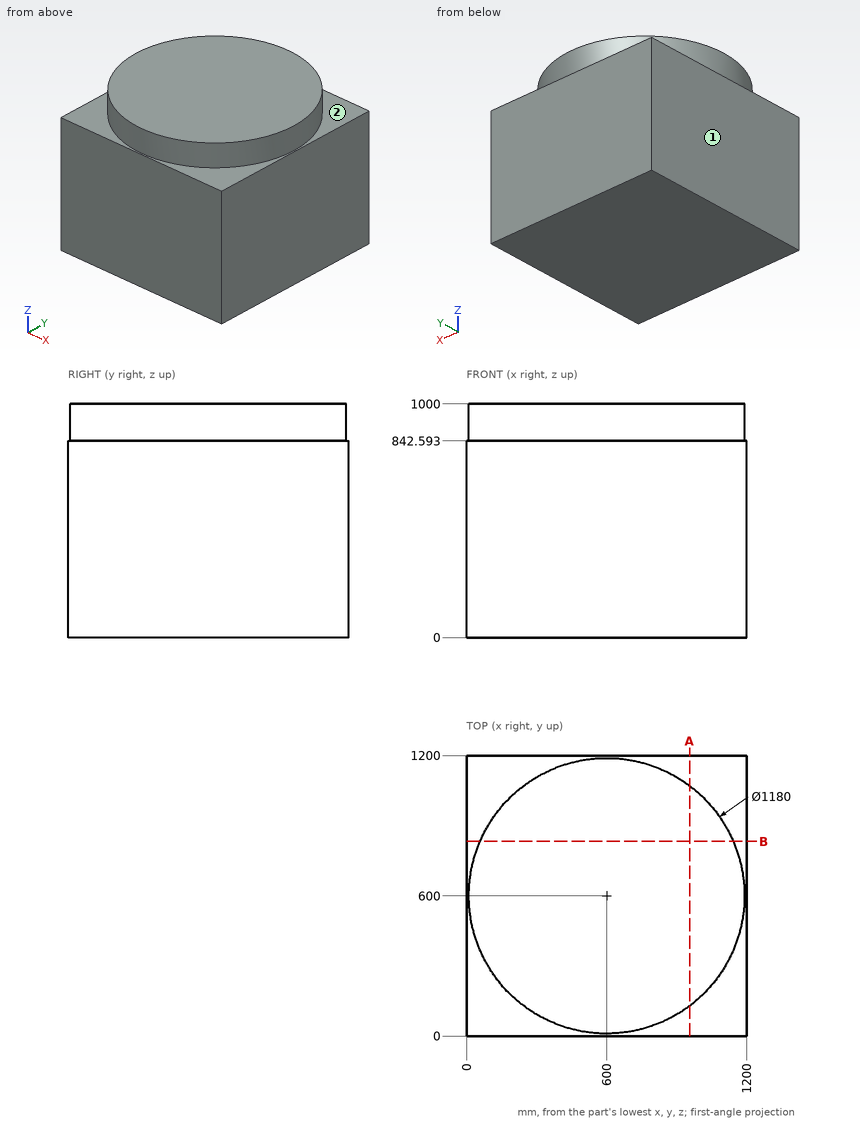
Answer from the drawing. Dimensions are ordinates in mm from the lowest x, y and z of the part. A direction names the side the tool comes from. Give positions to 0.01 mm unless a question says otherwise; leave off trailing zeros. Order: outer loops, then holes, each group sorted by start corner. A loop starts at its lowest first (then second) coordinate and runs counter-clockwise, first axis right, second up. Notation, with made-up numbers: (52.5, 88) -> (73.5, 88) arc R35 cw to (73.5, 121) -> close; hole circle Ø6 at (40.5, -9). An arc over 180 degrees is marked (long way). One line per item, written item: value. Start each with the question number.
(1) A flat-ended cylindrical pin translates along its axis: P1, Ø6, axis at x = 133, z = 895, coming from the -Y side. Find the tip coordinate at first contact, or state that the pin passes through.
(2) The part is cut by section A-A (x = 955.5). Determine the outline of the cut face in (y, z).
(3) The part is cut by section B-B (y = 832.5). Determine the outline of the cut face in (x, z).
(4) Straight lines are drawn through the part: L1, parallel to Z at x = 141, y = 125; L2, parallel to X at y = 234, z = 948 (1 decimal); L3, parallel to X at y = 208, z = 925. For each, find the intervals that lie inside material, in ascending order.
(5) A tool of negligible diameter and unlimited length cuts with its end or side. For the marked faces 1 and 2, from which of +Z, -Z, +X, -X, +Y, -Y can it reach the whole face along a straight path? Write none if from no direction.
Taken from the geometry:
1. P1: y = 235.58
2. outline: (0, 0) -> (1200, 0) -> (1200, 842.59) -> (1070.87, 842.59) -> (1070.87, 1000) -> (129.13, 1000) -> (129.13, 842.59) -> (0, 842.59) -> close
3. outline: (0, 0) -> (1200, 0) -> (1200, 842.59) -> (1142.26, 842.59) -> (1142.26, 1000) -> (57.74, 1000) -> (57.74, 842.59) -> (0, 842.59) -> close
4. L1: 0 to 842.59
4. L2: 137.2 to 1062.8
4. L3: 159.05 to 1040.95
5. face 1: +Z, -Z, -X, +Y, -Y
5. face 2: +Z
